```python
from build123d import *

# Parameters (mm, degrees)
SKETCH1_W           = 190
SKETCH1_H           = 110
SKETCH1_W_2         = 180
SKETCH1_H_2         = 100
BOSS_EXTRUDE1_DEPTH = 60
SKETCH2_W           = 110
SKETCH2_H           = 5
BOSS_EXTRUDE2_DEPTH = 190
SKETCH3_W           = 25
SKETCH3_H           = 20
CUT_EXTRUDE1_DEPTH  = 60


with BuildPart() as part:
    # Sketch1 → Boss-Extrude1 (new body)
    with BuildSketch(Plane(origin=(0, 0, 0), x_dir=(1, 0, 0), z_dir=(0, 1, 0))):
        with Locations((90, 50)):
            Rectangle(SKETCH1_W, SKETCH1_H)
        with Locations((90, 50)):
            Rectangle(SKETCH1_W_2, SKETCH1_H_2, mode=Mode.SUBTRACT)
    extrude(amount=BOSS_EXTRUDE1_DEPTH)

    # Sketch2 → Boss-Extrude2 (add)
    with BuildSketch(Plane(origin=(185, 0, 0), x_dir=(0, 0, -1), z_dir=(1, 0, 0))):
        with Locations((50, 2.5)):
            Rectangle(SKETCH2_W, SKETCH2_H)
    extrude(amount=-BOSS_EXTRUDE2_DEPTH)

    # Sketch3 → Cut-Extrude1 (cut)
    with BuildSketch(Plane(origin=(0, 0, -105), x_dir=(-1, 0, 0), z_dir=(0, 0, -1))):
        with Locations((-152.5, 15)):
            Rectangle(SKETCH3_W, SKETCH3_H)
    extrude(amount=-CUT_EXTRUDE1_DEPTH, mode=Mode.SUBTRACT)


solid = part.part
```
Work out the finished part from the listing and answer in its coordinate system (mm). A direction names the side the tool comes from. Coordinates: 2 decimals unless noted, no trailing zeros. Loops run counter-clockwise (first coordinate to the right, second up) from the corner with the lowest first, then second, coordinate; pieces in that order, holes last.
1) Section D-D (x = 75.5) is taken. Give the vertices of the cut face in (y, z), plus the area to 3 significant figures.
Results:
outline: (0, -105) - (60, -105) - (60, -100) - (5, -100) - (5, 0) - (60, 0) - (60, 5) - (0, 5) - close
area: 1,100 mm2
2) Section A-A (x = 147.5) is taken. Give the vertices of the cut face in (y, z).
Results:
outline: (0, -105) - (5, -105) - (5, 0) - (60, 0) - (60, 5) - (0, 5) - close; (25, -105) - (60, -105) - (60, -100) - (25, -100) - close
3) Section C-C (y = 44) is taken. Give the vertices of the cut face in (x, z), plus the area to 3 significant figures.
Results:
outline: (-5, -105) - (185, -105) - (185, 5) - (-5, 5) - close; hole (0, -100) - (180, -100) - (180, 0) - (0, 0) - close
area: 2,900 mm2
4) Consider probe 1 along Z at (x, y) = (87, 39); probe 2 along X at (y, z) = (54, -59); probe 3 along Y at (x, z) = (83, -53.5). Determine where each line is inside the solid, lowest interval first.
Results:
probe 1: z = -105 to -100, 0 to 5
probe 2: x = -5 to 0, 180 to 185
probe 3: y = 0 to 5
5) A flat-ended cylindrical pin translates along its axis: pin 1 (10 mm diameter, centred on x = 67, z = -89.5, fed in from +Y). Find the tip coordinate at first contact, or state that the pin passes through.
Results:
pin 1: stops at y = 5
6) Section B-B (z = -35.5) is taken. Give the vertices of the cut face in (x, y), plus the area to 3 significant figures.
Results:
outline: (-5, 0) - (185, 0) - (185, 60) - (180, 60) - (180, 5) - (0, 5) - (0, 60) - (-5, 60) - close
area: 1,500 mm2
7) For a pull along X with two mould halves and no side action, classify faces 1 (the flat face through (-5, 30, -49)), 2 (the flat face through (185, 30, -49)), 3 (the flat face through (0, 32, -49)), 4 (the flat face through (83, 60, 3)) as +X half, -X half, draft (parallel to the pull), parting line (faces both ways), or undercut.
Results:
face 1: -X half
face 2: +X half
face 3: undercut
face 4: draft
8) For faces 5 (the flat face through (153, 25, -103)), 6 (the flat face through (89, 0, -51)), 7 (the flat face through (89, 32, 0)), determine the directions among +Z, -Z, +X, -X, +Y, -Y from which every point of the face is accessible in a straight line to the end or side of a thin tool.
Results:
face 5: -Z
face 6: +Z, -Z, +X, -X, -Y
face 7: +Y
